The model under review builds one solid part; all positions refer to its coordinate system, in mm. A direction names the side the tool comes from. Round coordinates to 2 decimals unless told otherwise and drop trailing zeros. Loops run counter-clockwise (first coordinate to the right, second up) from the corner with the lowest first, then second, coordinate; pieces in that order, holes last. Notation, with made-up numbers: (27.5, 75) -> (71.5, 75) arc R21 cw to (71.5, 114) -> close; hole circle Ø8 at (77, 46). An arc over 180 degrees is marked (long way). Return JSON: item names as keys, results as strings. Group by question number.
```python
from build123d import *

# Parameters (mm, degrees)
SKETCH_1_R      = 4
EXTRUDE_1_DEPTH = 2.5
SKETCH_3_W      = 15
SKETCH_3_H      = 1
EXTRUDE_2_DEPTH = 0.2


with BuildPart() as part:
    # Эскиз1 → Бобышка-Вытянуть1 (new body)
    with BuildSketch(Plane(origin=(0, 0, 0), x_dir=(1, 0, 0), z_dir=(0, 1, 0))):
        with Locations(Location((0, 0, 0), (0, 0, 270))):
            Circle(SKETCH_1_R)
    extrude(amount=EXTRUDE_1_DEPTH)

    # Эскиз2 → Повернуть1 (revolve)
    with BuildSketch(Plane.XY):
        with BuildLine():
            Line((-2.5, 2.5), (0, 2.5))
            Line((0, 2.5), (0, 5))
            ThreePointArc((0, 5), (-1.767766953, 4.267766953), (-2.5, 2.5))
        make_face()
    revolve(axis=Axis((0, 0, 0), (0, 1, 0)))

    # Эскиз3 → Бобышка-Вытянуть2 (add)
    with BuildSketch(Plane(origin=(0, 0, 0), x_dir=(1, 0, 0), z_dir=(0, 1, 0))):
        with Locations((0, 2)):
            Rectangle(SKETCH_3_W, SKETCH_3_H)
        Rectangle(SKETCH_3_W, SKETCH_3_H)
        with Locations((0, -2)):
            Rectangle(SKETCH_3_W, SKETCH_3_H)
    extrude(amount=EXTRUDE_2_DEPTH)


solid = part.part
```
1. For P1, Ø1.1, axis at x = -5, z = 0, coming from the +Y side; P2, Ø1, axis at y = 1.5, z = -1, coming from the +X side; P3, Ø1.5, axis at y = 2, z = 1, coming from the -X side, all flat-tipped, find the tip position at first contact; note any pin that passes through.
2. We need section A-A, the plane x = -5. Write out the cut boundary in (y, z).
3. We need section C-C, the plane x = -1.5. Write out the cut boundary in (y, z), then the cut area to 3 significant figures.
4. We need section D-D, the plane y = 0.85. Write out the cut boundary in (x, z), then the cut area to 3 significant figures.
5. We need section B-B, the plane z = 0. Write out the cut boundary in (x, y).
6. Wall thickness on line 1 (Z direction, x = -1.5, y = 1.05); line 2 (Y direction, x = -1.75, z = 2); line 3 (X direction, y = 0.4, z = 0): over which ranges is each line inside the solid? List them lowest first.
7. Tool access review of faces 1 (the face through (2, 2.5, 2)), 2 (the face through (5, 0.2, 2)), 3 (the face through (-5, 0.2, 2)): name each direction out of +Z, -Z, +X, -X, +Y, -Y from which nothing blocks a thin tool from reaching the whole face with its end or side.
Check sheet entries:
{
 "1": {"P1": "stops at y = 0.2", "P2": "stops at x = 3.97", "P3": "stops at x = -3.99"},
 "2": {"outline": "(0, -2.5) -> (0.2, -2.5) -> (0.2, -1.5) -> (0, -1.5) -> close; (0, -0.5) -> (0.2, -0.5) -> (0.2, 0.5) -> (0, 0.5) -> close; (0, 1.5) -> (0.2, 1.5) -> (0.2, 2.5) -> (0, 2.5) -> close"},
 "3": {"outline": "(0, -3.71) -> (2.5, -3.71) -> (2.5, -2) arc R2 ccw to (2.5, 2) -> (2.5, 3.71) -> (0, 3.71) -> close", "area": "24.8 mm²"},
 "4": {"outline": "circle Ø8 at (0, 0)", "area": "50.3 mm²"},
 "5": {"outline": "(-7.5, 0) -> (7.5, 0) -> (7.5, 0.2) -> (4, 0.2) -> (4, 2.5) -> (2.5, 2.5) arc R2.5 ccw to (-2.5, 2.5) -> (-4, 2.5) -> (-4, 0.2) -> (-7.5, 0.2) -> close"},
 "6": {"line 1": "z = -3.71 to 3.71", "line 2": "y = 0 to 2.5", "line 3": "x = -4 to 4"},
 "7": {"face 1": "+Y", "face 2": "+Z, +X, +Y", "face 3": "+Z, -X, +Y"}
}
